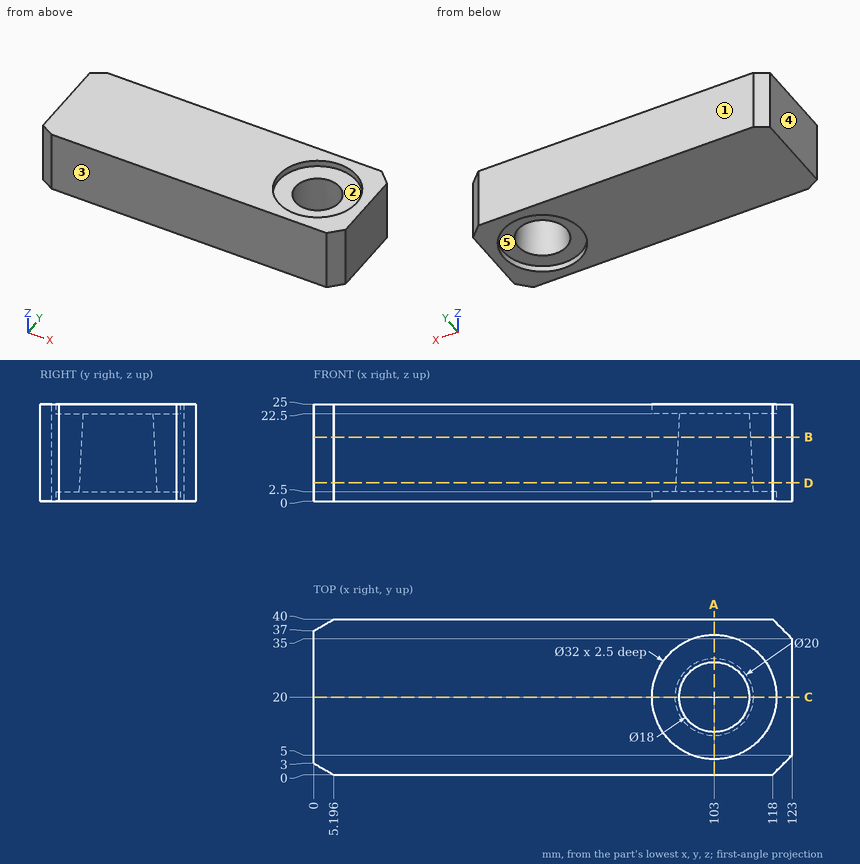
Design review of the part shown in the three views and the two pictorial views. Dimensions are in mm from the part's minimum x, y and z. A direction names the side the tool comes from. Give positions to 0.01 mm unless a question says otherwise; leave off trailing zeros. Order: outer loops, then holes, each group sorted by start corner. A loop starts at its lowest first (then second) coordinate and runs counter-clockwise, first axis right, second up. Notation, with made-up numbers: (49, 42.5) -> (96, 42.5) arc R13 ccw to (96, 63.5) -> close; hole circle Ø10 at (-10, 22.25). An arc over 180 degrees is marked (long way). Write each question's results on one line, items separated by ' | '. Start each with the question number.
Q1. Add section C-C on y = 20. Give the boundary of the cut face in (x, z), and give its area (4 significant figures).
Q2. Add section A-A on x = 103. Give the boundary of the cut face in (y, z), and give its area (3 significant figures).
Q3. Add section B-B on z = 16.5. Give the boundary of the cut face in (x, y), and give its area (3 significant figures).
Q4. Wall thickness on L1, parallel to Y at x = 103, z = 23.75; L2, parallel to X at y = 15.5, z = 4.75; L3, parallel to X at y = 18, z = 6.5: over which ranges is each line inside the solid? List them lowest first. Write a range as from..to.
Q5. Machinability: for the marked faces 4 and 5, which of the approach directions +Z, -Z, +X, -X, +Y, -Y give a long, thin tool a straight path to every point of the face, cutting with its end or side? Answer none if there is none.
Q6. Mouldability with a two-part tool opening along Y and no side actions: class the marked faces 1, 2 and 3 as +Y half, -Y half, draft (parallel to the pull), parting line (faces both ways), or undercut.
Q7. For pin 1 (5 mm diameter, centred on x = 94.5, y = 15, fed in from +Z), flat-tipped, find the tip position at first contact; note if it passes through.
Q8. Add section D-D on z = 4.75. Give the boundary of the cut face in (x, y) (1 decimal).
Found:
1) outline: (0, 0) -> (87, 0) -> (87, 2.5) -> (93, 2.5) -> (94, 22.5) -> (87, 22.5) -> (87, 25) -> (0, 25) -> close; (112, 22.5) -> (113, 2.5) -> (119, 2.5) -> (119, 0) -> (123, 0) -> (123, 25) -> (119, 25) -> (119, 22.5) -> close | area: 2,535 mm2
2) outline: (0, 0) -> (4, 0) -> (4, 2.5) -> (10, 2.5) -> (11, 22.5) -> (4, 22.5) -> (4, 25) -> (0, 25) -> close; (29, 22.5) -> (30, 2.5) -> (36, 2.5) -> (36, 0) -> (40, 0) -> (40, 25) -> (36, 25) -> (36, 22.5) -> close | area: 460 mm2
3) outline: (0, 3) -> (5.2, 0) -> (118, 0) -> (123, 5) -> (123, 35) -> (118, 40) -> (5.2, 40) -> (0, 37) -> close; hole circle Ø18.6 at (103, 20) | area: 4,610 mm2
4) L1: y = 0..4, 36..40 | L2: x = 0..94.2, 111.8..123 | L3: x = 0..93.41, 112.59..123
5) face 4: +Z, -Z, -X, +Y, -Y | face 5: -Z
6) face 1: +Y half | face 2: undercut | face 3: -Y half
7) pin 1: stops at z = 22.5
8) outline: (0, 3) -> (5.2, 0) -> (118, 0) -> (123, 5) -> (123, 35) -> (118, 40) -> (5.2, 40) -> (0, 37) -> close; hole circle Ø19.8 at (103, 20)
